Source: CAD feature listing. Evaluate the final solid. Frame: model axes, mm. A direction names the side the tool comes from. Round coordinates to 2 decimals unless told otherwise and drop trailing zeros. Write each loop counter-clockwise with the first axis right and the second up, starting at its lowest first coordinate (ties: lowest second). Pieces come first, ordered by that corner, then holes. Notation, with made-up numbers: M 77,-33.5 L 122,-33.5 A24 ccw 122,0.5 Z; hole C -12,62.25 d9. An arc over 180 degrees is marked long. Use a Markdown table: item, result.
```python
from build123d import *

# Parameters (mm, degrees)
SKETCH1_W            = 107.95
SKETCH1_H            = 101.6
BOSS_EXTRUDE1_DEPTH  = 2.54
SKETCH17_W           = 107.95
SKETCH17_H           = 2.54
BOSS_EXTRUDE11_DEPTH = 10.16
SKETCH20_W           = 111.76
SKETCH20_H           = 2.54
BOSS_EXTRUDE12_DEPTH = 10.16
SKETCH21_W           = 118.11
SKETCH21_H           = 2.54
BOSS_EXTRUDE13_DEPTH = 10.16
SKETCH22_W           = 121.92
SKETCH22_H           = 2.54
BOSS_EXTRUDE14_DEPTH = 10.16
SKETCH26_W           = 128.27
SKETCH26_H           = 121.92
BOSS_EXTRUDE18_DEPTH = 20.32
FILLET9_R            = 8.382
FILLET10_R           = 8.382
FILLET11_R           = 8.382
SKETCH28_W           = 101.6
SKETCH28_H           = 1.778
BOSS_EXTRUDE21_DEPTH = 25.4
SKETCH29_W           = 1.778
SKETCH29_H           = 88.9
BOSS_EXTRUDE22_DEPTH = 25.4
FILLET21_R           = 8.382
SKETCH30_W           = 101.6
SKETCH30_H           = 1.778
BOSS_EXTRUDE23_DEPTH = 25.4
SKETCH31_W           = 1.778
SKETCH31_H           = 101.6
BOSS_EXTRUDE24_DEPTH = 25.4
SKETCH32_R           = 1.524
CUT_EXTRUDE1_DEPTH   = 3.556
FILLET22_R           = 6.35
SKETCH34_W           = 2.376451265
SKETCH34_H           = 0.450830227
BOSS_EXTRUDE26_DEPTH = 0.762
BOSS_EXTRUDE27_DEPTH = 0.762
BOSS_EXTRUDE28_DEPTH = 0.762
SKETCH37_W           = 1.40164535
SKETCH37_H           = 0.295981153
BOSS_EXTRUDE29_DEPTH = 0.762
SKETCH38_W           = 0.721341472
SKETCH38_H           = 0.249868222
BOSS_EXTRUDE30_DEPTH = 0.762
SKETCH4_R            = 1.27
SKETCH4_R_2          = 0.762
BOSS_EXTRUDE31_DEPTH = 19.05
SKETCH40_R           = 1.524
CUT_EXTRUDE2_DEPTH   = 3.556
SKETCH42_W           = 29.21
SKETCH42_H           = 12.7
CUT_EXTRUDE3_DEPTH   = 3.556
SKETCH43_R           = 1.27
CUT_EXTRUDE4_DEPTH   = 2.54


with BuildPart() as part:
    # Sketch1 → Boss-Extrude1 (new body)
    with BuildSketch(Plane(origin=(0, 0, 0), x_dir=(1, 0, 0), z_dir=(0, 1, 0))):
        with Locations((-9.276565374, 13.725713086)):
            Rectangle(SKETCH1_W, SKETCH1_H)
    extrude(amount=BOSS_EXTRUDE1_DEPTH)

    # Sketch17 → Boss-Extrude11 (add)
    with BuildSketch(Plane(origin=(0, 0, -64.525713086), x_dir=(-1, 0, 0), z_dir=(0, 0, -1))):
        with Locations((9.276565374, 1.27)):
            Rectangle(SKETCH17_W, SKETCH17_H)
    extrude(amount=BOSS_EXTRUDE11_DEPTH)

    # Sketch20 → Boss-Extrude12 (add)
    with BuildSketch(Plane(origin=(44.698434626, 0, 0), x_dir=(0, 0, -1), z_dir=(1, 0, 0))):
        with Locations((18.805713086, 1.27)):
            Rectangle(SKETCH20_W, SKETCH20_H)
    extrude(amount=BOSS_EXTRUDE12_DEPTH)

    # Sketch21 → Boss-Extrude13 (add)
    with BuildSketch(Plane.XY.offset(37.074286914)):
        with Locations((-4.196565374, 1.27)):
            Rectangle(SKETCH21_W, SKETCH21_H)
    extrude(amount=BOSS_EXTRUDE13_DEPTH)

    # Sketch22 → Boss-Extrude14 (add)
    with BuildSketch(Plane.ZY.offset(63.251565374)):
        with Locations((-13.725713086, 1.27)):
            Rectangle(SKETCH22_W, SKETCH22_H)
    extrude(amount=BOSS_EXTRUDE14_DEPTH)

    # Sketch26 → Boss-Extrude18 (add)
    with BuildSketch(Plane(origin=(0, 2.54, 0), x_dir=(1, 0, 0), z_dir=(0, 1, 0))):
        with Locations((-9.276565374, 13.725713086)):
            Rectangle(SKETCH26_W, SKETCH26_H)
        Polygon((42.711561077, -45.456286914), (-66.807565374, -45.456286914), (-71.633565374, -40.630286914), (-71.633565374, -37.536996118), (-71.633565374, 66.303713086), (-71.633565374, 68.081713086), (-66.807565374, 72.907713086), (-62.278091081, 72.907713086), (48.254434626, 72.907713086), (53.080434626, 68.081713086), (53.080434626, -38.852286914), (53.080434626, -40.630286914), (48.254434626, -45.456286914), align=None, mode=Mode.SUBTRACT)
    extrude(amount=BOSS_EXTRUDE18_DEPTH)

    # Fillet9
    fillet9_edges = [part.edges().sort_by_distance(p)[0] for p in [
        (-73.411565374, 11.43, 47.234286914),
    ]]
    fillet(fillet9_edges, radius=FILLET9_R)

    # Fillet10
    fillet10_edges = [part.edges().sort_by_distance(p)[0] for p in [
        (54.858434626, 11.43, 47.234286914),
    ]]
    fillet(fillet10_edges, radius=FILLET10_R)

    # Fillet11
    fillet11_edges = [part.edges().sort_by_distance(p)[0] for p in [
        (-73.411565374, 11.43, -74.685713086),
    ]]
    fillet(fillet11_edges, radius=FILLET11_R)

    # Sketch28 → Boss-Extrude21 (add)
    with BuildSketch(Plane(origin=(0, 2.54, 0), x_dir=(1, 0, 0), z_dir=(0, 1, 0))):
        with Locations((-8.643546278, -44.567286914)):
            Rectangle(SKETCH28_W, SKETCH28_H)
    extrude(amount=BOSS_EXTRUDE21_DEPTH)

    # Sketch29 → Boss-Extrude22 (add)
    with BuildSketch(Plane(origin=(0, 2.54, 0), x_dir=(1, 0, 0), z_dir=(0, 1, 0))):
        with Locations((52.191434626, 16.003984914)):
            Rectangle(SKETCH29_W, SKETCH29_H)
    extrude(amount=BOSS_EXTRUDE22_DEPTH)

    # Fillet21
    fillet21_edges = [part.edges().sort_by_distance(p)[0] for p in [
        (54.858434626, 11.43, -74.685713086),
    ]]
    fillet(fillet21_edges, radius=FILLET21_R)

    # Sketch30 → Boss-Extrude23 (add)
    with BuildSketch(Plane(origin=(0, 2.54, 0), x_dir=(1, 0, 0), z_dir=(0, 1, 0))):
        with Locations((-10.117650569, 72.018713086)):
            Rectangle(SKETCH30_W, SKETCH30_H)
    extrude(amount=BOSS_EXTRUDE23_DEPTH)

    # Sketch31 → Boss-Extrude24 (add)
    with BuildSketch(Plane(origin=(0, 2.54, 0), x_dir=(1, 0, 0), z_dir=(0, 1, 0))):
        with Locations((-70.744565374, 17.281544489)):
            Rectangle(SKETCH31_W, SKETCH31_H)
    extrude(amount=BOSS_EXTRUDE24_DEPTH)

    # Sketch32 → Cut-Extrude1 (cut)
    with BuildSketch(Plane.XY.offset(47.234286914)):
        with Locations((-53.446124862, 13.468430173)):
            Circle(SKETCH32_R)
        with Locations((-48.874124862, 13.468430173)):
            Circle(SKETCH32_R)
        with Locations((-42.778124862, 13.468430173)):
            Circle(SKETCH32_R)
    extrude(amount=-CUT_EXTRUDE1_DEPTH, mode=Mode.SUBTRACT)

    # Fillet22
    fillet22_edges = [part.edges().sort_by_distance(p)[0] for p in [
        (-9.276565374, 0, 47.234286914),
        (-70.956534413, 0, 44.779255954),
        (54.858434626, 0, -13.725713086),
        (52.403403666, 0, 44.779255954),
        (-73.411565374, 0, -13.725713086),
        (-70.956534413, 0, -72.230682126),
        (-9.276565374, 0, -74.685713086),
        (52.403403666, 0, -72.230682126),
    ]]
    fillet(fillet22_edges, radius=FILLET22_R)

    # Sketch34 → Boss-Extrude26 (add)
    with BuildSketch(Plane.XY.offset(47.234286914)):
        with Locations((-48.746578478, 9.905961703)):
            Rectangle(SKETCH34_W, SKETCH34_H)
    extrude(amount=BOSS_EXTRUDE26_DEPTH)

    # Sketch35 → Boss-Extrude27 (add)
    with BuildSketch(Plane.XY.offset(47.234286914)):
        Polygon((-53.675043022, 11.10789921), (-53.182867877, 11.10789921), (-53.182867877, 10.345394629), (-52.415207401, 10.345394629), (-52.415207401, 9.941250014), (-53.182867877, 9.941250014), (-53.182867877, 9.28546766), (-53.675043022, 9.28546766), (-53.675043022, 9.941250014), (-54.332901543, 9.941250014), (-54.332901543, 10.345394629), (-53.675043022, 10.345394629), align=None)
    extrude(amount=BOSS_EXTRUDE27_DEPTH)

    # Sketch36 → Boss-Extrude28 (add)
    with BuildSketch(Plane.XY.offset(47.234286914)):
        Polygon((-42.938376237, 10.774794696), (-42.938376237, 11.391124792), (-42.570939626, 11.391124792), (-42.570939626, 10.774794696), (-41.773582858, 10.774794696), (-41.773582858, 10.421472403), (-43.74903155, 10.421472403), (-43.74903155, 10.774794696), align=None)
    extrude(amount=BOSS_EXTRUDE28_DEPTH)

    # Sketch37 → Boss-Extrude29 (add)
    with BuildSketch(Plane.XY.offset(47.234286914)):
        with Locations((-42.779535982, 10.098380285)):
            Rectangle(SKETCH37_W, SKETCH37_H)
    extrude(amount=BOSS_EXTRUDE29_DEPTH)

    # Sketch38 → Boss-Extrude30 (add)
    with BuildSketch(Plane.XY.offset(47.234286914)):
        with Locations((-42.785601146, 9.583230105)):
            Rectangle(SKETCH38_W, SKETCH38_H)
    extrude(amount=BOSS_EXTRUDE30_DEPTH)

    # Sketch4 → Boss-Extrude31 (add)
    with BuildSketch(Plane(origin=(0, 2.54, 0), x_dir=(1, 0, 0), z_dir=(0, 1, 0))):
        with Locations((-36.327565374, 11.439713086)):
            Circle(SKETCH4_R)
        with Locations((-36.327565374, 11.439713086)):
            Circle(SKETCH4_R_2, mode=Mode.SUBTRACT)
        with Locations((28.188434626, 7.883713086)):
            Circle(SKETCH4_R)
        with Locations((28.188434626, 7.883713086)):
            Circle(SKETCH4_R_2, mode=Mode.SUBTRACT)
    extrude(amount=BOSS_EXTRUDE31_DEPTH)

    # Sketch40 → Cut-Extrude2 (cut)
    with BuildSketch(Plane.XY.offset(47.234286914)):
        with Locations((-37.012349316, 15.614831818)):
            Circle(SKETCH40_R)
        with Locations((-32.223462278, 15.614831818)):
            Circle(SKETCH40_R)
        with Locations((-37.012349316, 11.291329779)):
            Circle(SKETCH40_R)
        with Locations((-32.223462278, 11.291329779)):
            Circle(SKETCH40_R)
    extrude(amount=-CUT_EXTRUDE2_DEPTH, mode=Mode.SUBTRACT)

    # Sketch42 → Cut-Extrude3 (cut)
    with BuildSketch(Plane(origin=(54.858434626, 0, 0), x_dir=(0, 0, -1), z_dir=(1, 0, 0))):
        with Locations((41.538713086, 14.605)):
            Rectangle(SKETCH42_W, SKETCH42_H)
    extrude(amount=-CUT_EXTRUDE3_DEPTH, mode=Mode.SUBTRACT)

    # Sketch43 → Cut-Extrude4 (cut)
    with BuildSketch(Plane(origin=(0, 2.54, 0), x_dir=(1, 0, 0), z_dir=(0, 1, 0))):
        with Locations((-14.323930267, -5.830780993)):
            Circle(SKETCH43_R)
        with Locations((-52.423930267, -5.830780993)):
            Circle(SKETCH43_R)
        with Locations((-52.423930267, -38.850780993)):
            Circle(SKETCH43_R)
        with Locations((-14.323930267, -38.850780993)):
            Circle(SKETCH43_R)
    extrude(amount=-CUT_EXTRUDE4_DEPTH, mode=Mode.SUBTRACT)


solid = part.part
```
Q1. First-contact query: pin 1 Ø0.8 at (x, z) = (-42.5, 47.5) entering from +Y; pin 2 Ø1.1 at (x, y) = (53, 16) entering from -Z; pin 3 Ø4 at (x, y) = (16.5, 4) entering from +Z. Flat tips, straight axial feed; report the tip coordinate or a pass-through.
Results are:
| item | result |
|---|---|
| pin 1 | y = 22.86 |
| pin 2 | z = -72.18 |
| pin 3 | z = 47.22 |
Q2. Reachability of faces 4 (the cylindrical face through (-37.343, 9.804, 45.481)), 5 (the flat face through (-9, 25, 45.456)), 6 (the flat face through (53.08, 13, 34)), 7 (the flat face through (53, 8.255, -41)) from +Z, -Z, +X, -X, +Y, -Y: full face, straight path, thin tool, end or side. Return the list, or none.
Results are:
| item | result |
|---|---|
| face 4 | +Z |
| face 5 | +Z, +X, -X, +Y |
| face 6 | +Y |
| face 7 | +X |
Q3. Mould query, pull axis X, two halves, no side actions, for faces 1 (the flat face through (-10, 14, -74.686)), 2 (the cylindrical face through (-71.021, 14.721, 44.714)), 3 (the flat face through (-71.634, 13, 37)). Classes: +X half, -X half, draft (parallel to the pull), parting line (faces both ways), or undercut.
Results are:
| item | result |
|---|---|
| face 1 | draft |
| face 2 | -X half |
| face 3 | undercut |
Q4. Section C-C on x = -63.5. Return loops of the section in (y, z), plus the area to 3 significant figures.
Results are:
| item | result |
|---|---|
| outline | M 0,-68.34 A6.35 ccw 6.35,-74.69 L 22.86,-74.69 L 22.86,-72.91 L 2.54,-72.91 L 2.54,45.46 L 22.86,45.46 L 22.86,47.23 L 6.35,47.23 A6.35 ccw 0,40.88 Z |
| area | 365 mm^2 |
Q5. Section A-A on y = 25.75. Return loops of the section in (x, z), plus the area to 3 significant figures.
Results are:
| item | result |
|---|---|
| outline | M -71.63,-68.08 L -69.86,-68.08 L -69.86,33.52 L -71.63,33.52 Z; M -60.92,-72.91 L 40.68,-72.91 L 40.68,-71.13 L -60.92,-71.13 Z; M -59.44,43.68 L 42.16,43.68 L 42.16,45.46 L -59.44,45.46 Z; M 51.3,-60.45 L 53.08,-60.45 L 53.08,28.45 L 51.3,28.45 Z |
| area | 700 mm^2 |
Q6. Line query: L1, parallel to Z at x = -2, y = 12.75; L2, parallel to X at y = 19.5, z = -13.5; L3, parallel to X at y = 20.25, z = 36.5. Output: solid intervals per line, ascending.
Results are:
| item | result |
|---|---|
| L1 | -74.69 to -71.13, 43.68 to 47.23 |
| L2 | -73.41 to -69.86, 51.3 to 54.86 |
| L3 | -73.41 to -71.63, 53.08 to 54.86 |
Q7. Section D-D on z = 12. Return loops of the section in (x, y).
Results are:
| item | result |
|---|---|
| outline | M -73.41,6.35 A6.35 ccw -67.06,0 L 48.51,0 A6.35 ccw 54.86,6.35 L 54.86,22.86 L 53.08,22.86 L 53.08,27.94 L 51.3,27.94 L 51.3,2.54 L -69.86,2.54 L -69.86,27.94 L -71.63,27.94 L -71.63,22.86 L -73.41,22.86 Z |
Q8. Section B-B on z = -28.5. Return loops of the section in (x, y) (3 decimals).
Results are:
| item | result |
|---|---|
| outline | M -73.412,6.35 A6.35 ccw -67.062,0 L 48.508,0 A6.35 ccw 54.858,6.35 L 54.858,8.255 L 51.302,8.255 L 51.302,2.54 L -69.856,2.54 L -69.856,27.94 L -71.634,27.94 L -71.634,22.86 L -73.412,22.86 Z; M 51.302,20.955 L 54.858,20.955 L 54.858,22.86 L 53.08,22.86 L 53.08,27.94 L 51.302,27.94 Z |
